Can you work these out from the drawing? Everything is in mm from the part's minimum corner. Round coordinates to 2 decimals unless told otherwise and drop trailing zeros. Loops run counter-clockwise (first coordinate to the right, second up) from the corner with the lowest first, then second, coordinate; pieces in that order, holes last. Notation, with made-up numbers: M 75,35.25 L 81,35.25 A23 cw 81,72.25 Z; hole C 38.25,47.25 d6. An arc over 180 degrees is marked long. Use a Markdown table: item, result.
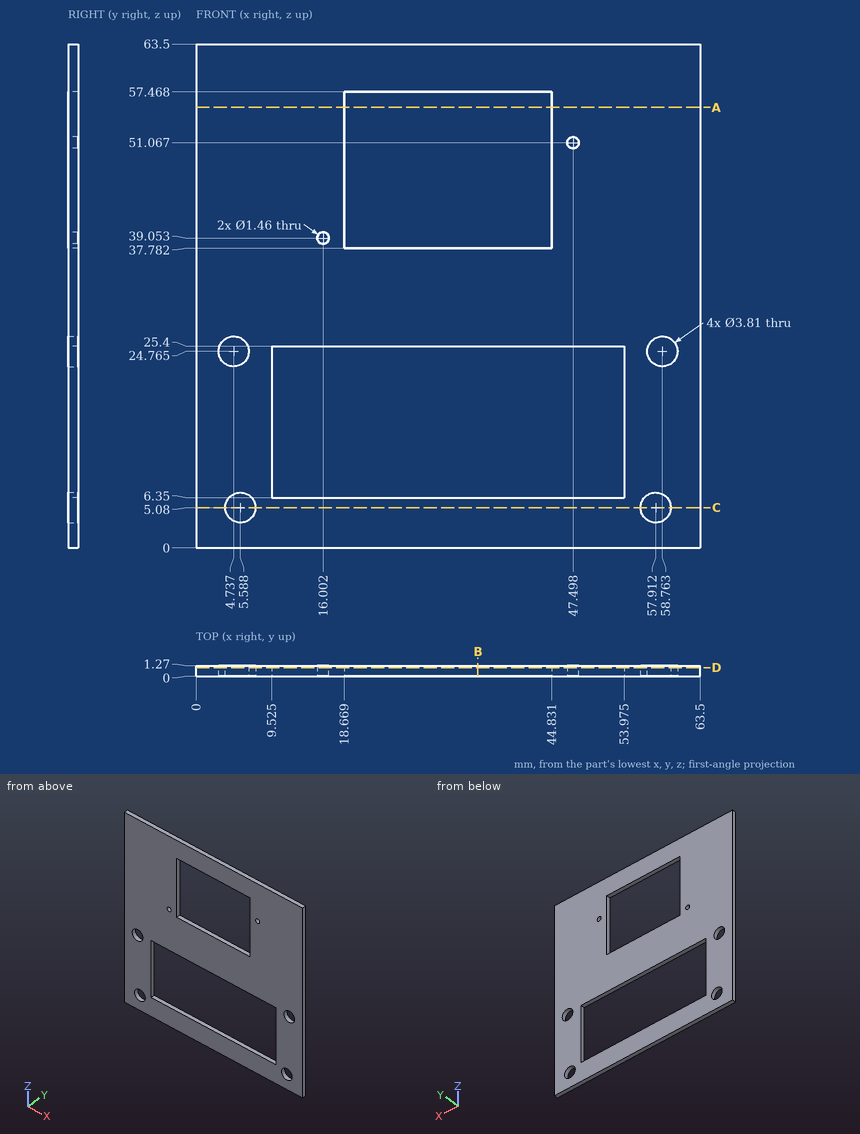
1. I need wall thicknesses on probe 1 along X at (y, z) = (0.4, 5.08); probe 2 along Z at (x, y) = (26, 0.7); probe 3 along Z at (x, y) = (45.5, 1.2). Which ranges of each line are inside material? Lowest first, please. Write a range as from..to.
Answer sheet:
| item | result |
|---|---|
| probe 1 | 0..3.68, 7.49..56.01, 59.82..63.5 |
| probe 2 | 0..6.35, 25.4..37.78, 57.47..63.5 |
| probe 3 | 0..6.35, 25.4..63.5 |
2. Imagine slicing it at D-D, the plane y = 1.05. State how many separate pieces and enclosed holes the cut face has, then the cut area to 3 significant figures.
Answer sheet:
| item | result |
|---|---|
| separate pieces | 1 |
| enclosed holes | 8 |
| area | 2,620 mm2 |
3. Imagine slicing it at A-A, the plane z = 55.5. Write out the boundary of the cut face in (x, y).
Answer sheet:
| item | result |
|---|---|
| outline | M 0,0 L 18.67,0 L 18.67,1.27 L 0,1.27 Z; M 44.83,0 L 63.5,0 L 63.5,1.27 L 44.83,1.27 Z |
4. Imagine slicing it at C-C, the plane z = 5.08. Write out the boundary of the cut face in (x, y).
Answer sheet:
| item | result |
|---|---|
| outline | M 0,0 L 3.68,0 L 3.68,1.27 L 0,1.27 Z; M 7.49,0 L 56.01,0 L 56.01,1.27 L 7.49,1.27 Z; M 59.82,0 L 63.5,0 L 63.5,1.27 L 59.82,1.27 Z |
5. Imagine slicing it at B-B, the plane x = 35.5. Write out the boundary of the cut face in (y, z).
Answer sheet:
| item | result |
|---|---|
| outline | M 0,0 L 1.27,0 L 1.27,6.35 L 0,6.35 Z; M 0,25.4 L 1.27,25.4 L 1.27,37.78 L 0,37.78 Z; M 0,57.47 L 1.27,57.47 L 1.27,63.5 L 0,63.5 Z |
